The drawing under review shows one solid part. Ordinate dimensions are in mm from its lowest x, y, z. A direction names the side the tool comes from. Coordinates: 2 decimals unless noted, no trailing zeros. Write each loop counter-clockwise with the first axis right and the second up, starting at its lowest first coordinate (ties: lowest second). Pieces come first, ordered by that corner, then holes.
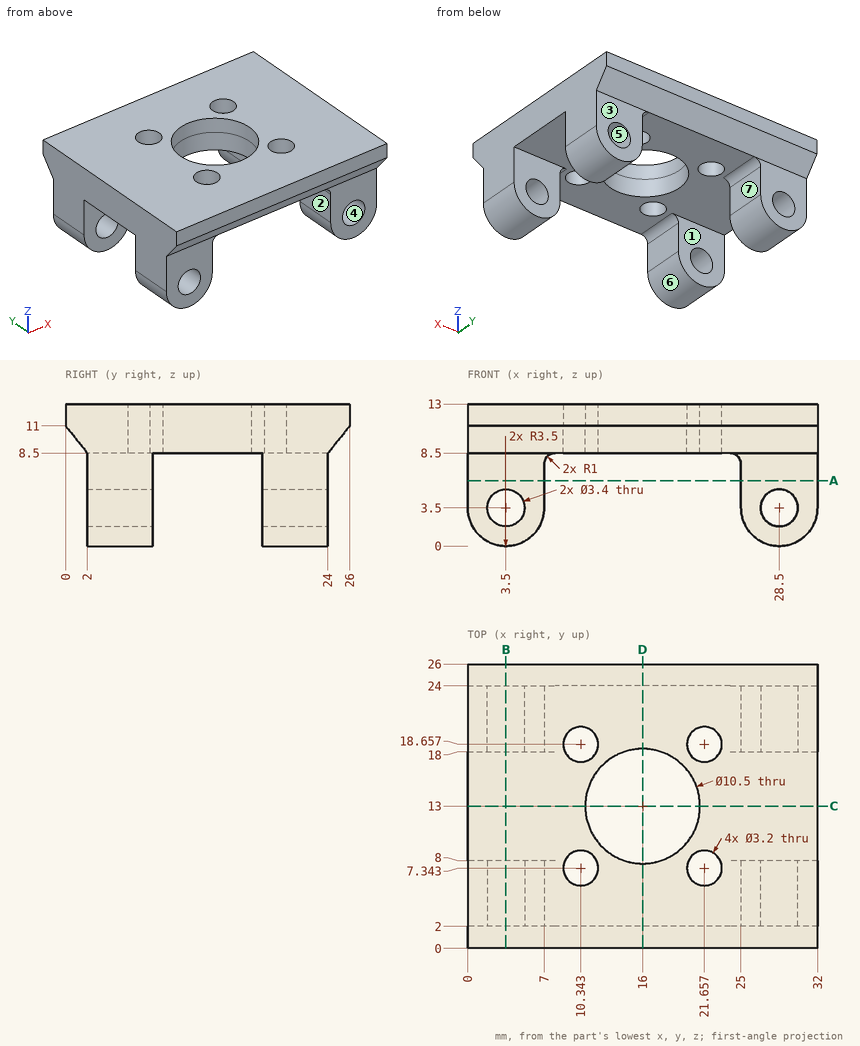
1) Consider section D-D (x = 16). Give the boundary of the cut face in (y, z).
2) The part is to be moulded in two halves that separate along Z. For the marked faces 4, 5, 6 and 7, say which applies: pulls with the +Z half, pulls with the -Z half, needs draft (parallel to the pull), parting line crosses it, or undercut.
3) Consider section A-A (z = 6). Give the boundary of the cut face in (x, y).
4) Consider section B-B (x = 3.5). Give the boundary of the cut face in (y, z), then the cut area to 3 significant figures.
5) Clearance check with flat-ended pins moving along their axes: P1, Ø2.5, axis at x = 26.5, z = 3, coming from the -Y side; P2, Ø3, axis at x = 17.5, y = 22.5, coming from the -Z side; P3, Ø4, axis at x = 3.5, z = 5.5, coming from the +Y side. State where each tip first meets the part, or that it passes through.
6) Tool access review of the marked faces 1, 2 and 3: name each direction out of +Z, -Z, +X, -X, +Y, -Y from which nothing blocks a thin tool from reaching the whole face with its end or side.
7) For L1, parallel to X at y = 22.5, z = 3.5; L2, parallel to Y at x = 3.5, z = 5.5; L3, parallel to Y at x = 16, z = 11.55, list the stretches that pass through material, from the lowest coordinate up.
8) Consider section C-C (y = 13). Give the boundary of the cut face in (x, z).
Results:
1. outline: (0, 11) - (2, 8.5) - (7.75, 8.5) - (7.75, 13) - (0, 13) - close; (18.25, 8.5) - (24, 8.5) - (26, 11) - (26, 13) - (18.25, 13) - close
2. face 4: undercut
2. face 5: undercut
2. face 6: pulls with the -Z half
2. face 7: needs draft
3. outline: (0, 2) - (7, 2) - (7, 8) - (0, 8) - close; (0, 18) - (7, 18) - (7, 24) - (0, 24) - close; (25, 2) - (32, 2) - (32, 8) - (25, 8) - close; (25, 18) - (32, 18) - (32, 24) - (25, 24) - close
4. outline: (0, 11) - (2, 8.5) - (2, 5.2) - (8, 5.2) - (8, 8.5) - (18, 8.5) - (18, 5.2) - (24, 5.2) - (24, 8.5) - (26, 11) - (26, 13) - (0, 13) - close; (2, 0) - (8, 0) - (8, 1.8) - (2, 1.8) - close; (18, 0) - (24, 0) - (24, 1.8) - (18, 1.8) - close
4. area: 173 mm2
5. P1: stops at y = 2
5. P2: stops at z = 8.5
5. P3: stops at y = 24
6. face 1: -Z, +X, -X
6. face 2: -Z, +Y, -Y
6. face 3: -Z, +X, -X, +Y
7. L1: x = 0 to 1.8, 5.2 to 7, 25 to 26.8, 30.2 to 32
7. L2: y = 2 to 8, 18 to 24
7. L3: y = 0 to 7.75, 18.25 to 26
8. outline: (0, 8.5) - (10.75, 8.5) - (10.75, 13) - (0, 13) - close; (21.25, 8.5) - (32, 8.5) - (32, 13) - (21.25, 13) - close
